Source: CAD feature listing. Evaluate the final solid. Frame: model axes, mm. A direction names the side the tool comes from. Round coordinates to 2 decimals unless told otherwise and drop trailing zeros. Write each loop counter-clockwise with the first axis right and the second up, starting at its lowest first coordinate (ties: lowest second). Pieces come first, ordered by that corner, then holes.
from build123d import *

# Parameters (mm, degrees)
ESQUISSE2_W             = 183
ESQUISSE2_H             = 133
BOSS_EXTRU_2_DEPTH      = 50
ESQUISSE3_W             = 50
ESQUISSE3_H             = 15
ENL_V_MAT_EXTRU_1_DEPTH = 50
CONG_1_R                = 5
ENL_V_MAT_EXTRU_3_DEPTH = 4
ENL_V_MAT_EXTRU_4_DEPTH = 4
ENL_V_MAT_EXTRU_5_DEPTH = 4


with BuildPart() as part:
    # Esquisse2 → Boss.-Extru.2 (new body)
    with BuildSketch(Plane.XY):
        Rectangle(ESQUISSE2_W, ESQUISSE2_H)
        Polygon((-85.996240602, -62.5), (-87.5, -62.5), (-87.5, 62.5), (87.5, 62.5), (87.5, -62.5), align=None, mode=Mode.SUBTRACT)
    extrude(amount=BOSS_EXTRU_2_DEPTH)

    # Esquisse3 → Enlèv. mat.-Extru.1 (cut)
    with BuildSketch(Plane(origin=(0, 66.5, 0), x_dir=(1, 0, 0), z_dir=(0, 1, 0))):
        with Locations((4, -42.5)):
            Rectangle(ESQUISSE3_W, ESQUISSE3_H)
    extrude(amount=-ENL_V_MAT_EXTRU_1_DEPTH, mode=Mode.SUBTRACT)

    # Congé1
    cong_1_edges = [part.edges().sort_by_distance(p)[0] for p in [
        (91.5, -66.5, 25),
        (91.5, 66.5, 25),
        (-91.5, 66.5, 25),
        (-91.5, -66.5, 25),
    ]]
    fillet(cong_1_edges, radius=CONG_1_R)

    # Esquisse6 → Enlèv. mat.-Extru.3 (cut)
    with BuildSketch(Plane(origin=(91.5, 0, 0), x_dir=(0, 0, -1), z_dir=(1, 0, 0))):
        Polygon((-50, 20.9), (-47, 20.9), (-47, 19.65), (-42.8, 19.65), (-42.8, 20.9), (-39, 20.9), (-39, 24.1), (-42.8, 24.1), (-42.8, 25.35), (-47, 25.35), (-47, 24.1), (-50, 24.1), align=None)
        Polygon((-50, -24.1), (-47, -24.1), (-47, -25.35), (-42.8, -25.35), (-42.8, -24.1), (-39, -24.1), (-39, -20.9), (-42.8, -20.9), (-42.8, -19.65), (-47, -19.65), (-47, -20.9), (-50, -20.9), align=None)
    extrude(amount=-ENL_V_MAT_EXTRU_3_DEPTH, mode=Mode.SUBTRACT)

    # Esquisse7 → Enlèv. mat.-Extru.4 (cut)
    with BuildSketch(Plane.ZY.offset(91.5)):
        Polygon((47, 20.9), (50, 20.9), (50, 24.1), (47, 24.1), (47, 25.35), (42.8, 25.35), (42.8, 24.1), (39, 24.1), (39, 20.9), (42.8, 20.9), (42.8, 19.65), (47, 19.65), align=None)
        Polygon((47, -24.1), (50, -24.1), (50, -20.9), (47, -20.9), (47, -19.65), (42.8, -19.65), (42.8, -20.9), (39, -20.9), (39, -24.1), (42.8, -24.1), (42.8, -25.35), (47, -25.35), align=None)
    extrude(amount=-ENL_V_MAT_EXTRU_4_DEPTH, mode=Mode.SUBTRACT)

    # Esquisse9 → Enlèv. mat.-Extru.5 (cut)
    with BuildSketch(Plane.XZ.offset(66.5)):
        Polygon((-49.1, 50), (-45.9, 50), (-45.9, 47), (-44.65, 47), (-44.65, 42.8), (-45.9, 42.8), (-45.9, 39), (-49.1, 39), (-49.1, 42.8), (-50.35, 42.8), (-50.35, 47), (-49.1, 47), align=None)
        Polygon((45.9, 50), (45.9, 47), (44.65, 47), (44.65, 42.8), (45.9, 42.8), (45.9, 39), (49.1, 39), (49.1, 42.8), (50.35, 42.8), (50.35, 47), (49.1, 47), (49.1, 50), align=None)
    extrude(amount=-ENL_V_MAT_EXTRU_5_DEPTH, mode=Mode.SUBTRACT)


solid = part.part
1) Reachability of faces 1 (the face through (-87.5, -1, 25)), 2 (the face through (-21, 65, 43)), 3 (the face through (90, 24.1, 41)), 4 (the face through (-44.65, -65, 45)) from +Z, -Z, +X, -X, +Y, -Y: full face, straight path, thin tool, end or side. Return the list, or none.
Taken from the geometry:
face 1: +Z, -Z
face 2: +Z, +Y
face 3: +Z, +X, -X
face 4: -Y
2) Section query B-B on y = 44.5. Return the cut outline in (x, z).
Taken from the geometry:
outline: (-91.5, 0) - (-87.5, 0) - (-87.5, 50) - (-91.5, 50) - close; (87.5, 0) - (91.5, 0) - (91.5, 50) - (87.5, 50) - close
3) Material intervals for line 1 (X direction, y = 47, z = 25.5); line 2 (Y direction, x = 9.5, z = 34); line 3 (Y direction, x = 17.5, z = 39), sorted ascending.
Taken from the geometry:
line 1: x = -91.5 to -87.5, 87.5 to 91.5
line 2: y = -66.5 to -62.5, 62.5 to 66.5
line 3: y = -66.5 to -62.5
4) Section query C-C on z = 18.5. Return the cut outline in (x, y), then the cut area to 3 significant figures.
Taken from the geometry:
outline: (-91.5, -61.5) arc R5 ccw to (-86.5, -66.5) - (86.5, -66.5) arc R5 ccw to (91.5, -61.5) - (91.5, 61.5) arc R5 ccw to (86.5, 66.5) - (-86.5, 66.5) arc R5 ccw to (-91.5, 61.5) - close; hole (-87.5, -62.5) - (87.5, -62.5) - (87.5, 62.5) - (-87.5, 62.5) - close
area: 2,440 mm2
5) Contact query for flat-ended pins moving along their axis: P1, Ø4.5, axis at x = -90.5, z = 44.5, coming from the -Y side; P2, Ø1.2, axis at x = 90, z = 46, coming from the +Y side; P3, Ø1.9, axis at x = -89, z = 40, coming from the +Y side. Output: stop coordinate, or through.
Taken from the geometry:
P1: stops at y = -66.18
P2: stops at y = 65.57
P3: stops at y = 66.25
6) Section query A-A on x = 15.5. Return the cut outline in (y, z).
Taken from the geometry:
outline: (-66.5, 0) - (-62.5, 0) - (-62.5, 50) - (-66.5, 50) - close; (62.5, 0) - (66.5, 0) - (66.5, 35) - (62.5, 35) - close
7) Pull-direction query (X, two-part tool) for faces 5 (the face through (50.35, -65, 45)), 6 (the face through (-90.07, -65, 25.35)), 7 (the face through (-90, 24.1, 41)); classes: released by +X, released by -X, zero draft, split by the parting line, or undercut.
Taken from the geometry:
face 5: undercut
face 6: released by -X
face 7: zero draft
